For this review, take the finished solid that the model builds, in its own axes (mm). Give positions to 0.01 mm unless a question says otherwise; leave off trailing zeros. Write each loop counter-clockwise with the first axis right and the second up, starting at its lowest first coordinate (ties: lowest second). Pieces come first, ordered by that corner, then holes.
1) For P1, Ø1, axis at y = 3.5, z = 78.5, coming from the -X side, flat-tipped, find the tip position at first contact; note if it passes through.
2) Wall thickness on line 1 along Z through (x, y) = (2.75, 0); line 2 along Z through (x, y) = (1.15, -1.5); line 3 along Z through (x, y) = (0.35, 2.75): over which ranges is each line inside the solid? List them lowest first.
3) We need section B-B on y = 0. Give the boundary of the cut face in (x, z) (1 decimal).
4) We need section C-C on x = 0.9. Give the boundary of the cut face in (y, z) (1 decimal).
5) We need section A-A on z = 76.2. Give the boundary of the cut face in (x, y) (1 decimal), and give its area (3 significant figures).
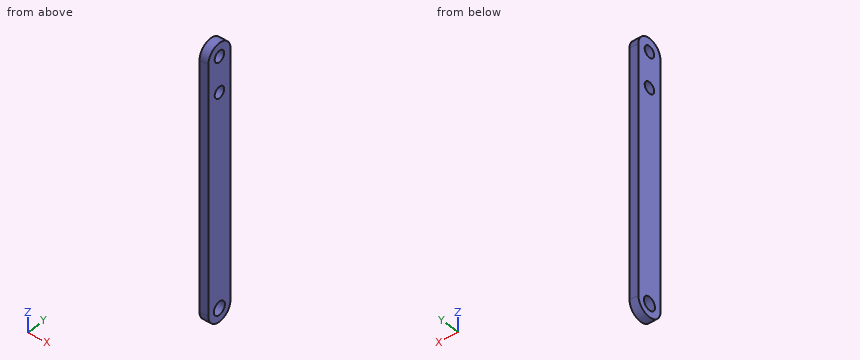
from build123d import *

# Parameters (mm, degrees)
F0_R     = 2.032
F0_R_2   = 2.38125
F1_DEPTH = 3.175


with BuildPart() as f1:
    # F0 (on Right) → F1 (new body)
    with BuildSketch(Plane.YZ):
        with BuildLine():
            Line((4.7625, 0), (4.7625, 88.9))
            ThreePointArc((4.7625, 88.9), (0, 93.6625), (-4.7625, 88.9))
            Line((-4.7625, 88.9), (-4.7625, 0))
            ThreePointArc((-4.7625, 0), (0, 4.7625), (4.7625, 0))
        make_face()
        with Locations((0, 76.2)):
            Circle(F0_R, mode=Mode.SUBTRACT)
        with Locations((0, 88.9)):
            Circle(F0_R, mode=Mode.SUBTRACT)
        with BuildLine():
            ThreePointArc((-4.7625, 0), (0, -4.7625), (4.7625, 0))
            ThreePointArc((4.7625, 0), (0, 4.7625), (-4.7625, 0))
        make_face()
        Circle(F0_R_2, mode=Mode.SUBTRACT)
    extrude(amount=F1_DEPTH)


solid = f1.part
Results list:
1. P1: stops at x = 0
2. line 1: z = -4.76 to -2.38, 2.38 to 74.17, 78.23 to 86.87, 90.93 to 93.66
2. line 2: z = -4.52 to -1.85, 1.85 to 74.83, 77.57 to 87.53, 90.27 to 93.42
2. line 3: z = -3.89 to 92.79
3. outline: (0, -4.8) - (3.2, -4.8) - (3.2, -2.4) - (0, -2.4) - close; (0, 2.4) - (3.2, 2.4) - (3.2, 74.2) - (0, 74.2) - close; (0, 78.2) - (3.2, 78.2) - (3.2, 86.9) - (0, 86.9) - close; (0, 90.9) - (3.2, 90.9) - (3.2, 93.7) - (0, 93.7) - close
4. outline: (-4.8, 0) arc R4.8 ccw to (4.8, 0) - (4.8, 88.9) arc R4.8 ccw to (-4.8, 88.9) - close; hole circle Ø4.8 at (0, 0); hole circle Ø4.1 at (0, 76.2); hole circle Ø4.1 at (0, 88.9)
5. outline: (0, -4.8) - (3.2, -4.8) - (3.2, -2) - (0, -2) - close; (0, 2) - (3.2, 2) - (3.2, 4.8) - (0, 4.8) - close
5. area: 17.3 mm2
